```python
from build123d import *

# Parameters (mm, degrees)
SKETCH1_W           = 57
SKETCH1_H           = 52
BOSS_EXTRUDE1_DEPTH = 4
SKETCH3_W           = 37
SKETCH3_H           = 37
BOSS_EXTRUDE2_DEPTH = 3
SKETCH4_W           = 37
SKETCH4_H           = 37
BOSS_EXTRUDE3_DEPTH = 3
SKETCH6_R           = 1.5
BOSS_EXTRUDE4_DEPTH = 10
SKETCH6_6_R         = 1.5
BOSS_EXTRUDE6_DEPTH = 10
SKETCH8_W           = 4
SKETCH8_H           = 22
CUT_EXTRUDE1_DEPTH  = 11


with BuildPart() as part:
    # Sketch1 → Boss-Extrude1 (new body)
    with BuildSketch(Plane.XY):
        Rectangle(SKETCH1_W, SKETCH1_H)
    extrude(amount=BOSS_EXTRUDE1_DEPTH)

    # Sketch3 → Boss-Extrude2 (add)
    with BuildSketch(Plane.XY.offset(4)):
        with Locations((0, 7.5)):
            Rectangle(SKETCH3_W, SKETCH3_H)
    extrude(amount=BOSS_EXTRUDE2_DEPTH)

    # Sketch4 → Boss-Extrude3 (add)
    with BuildSketch(Plane(origin=(0, 0, 0), x_dir=(-1, 0, 0), z_dir=(0, 0, -1))):
        with Locations((0, 7.5)):
            Rectangle(SKETCH4_W, SKETCH4_H)
    extrude(amount=BOSS_EXTRUDE3_DEPTH)

    # Sketch6 → Boss-Extrude4 (add)
    with BuildSketch(Plane.XY):
        with Locations((14.91830134, 22.543210914)):
            Circle(SKETCH6_R)
        with Locations((14.91830134, -7.514403638)):
            Circle(SKETCH6_R)
    extrude(amount=-BOSS_EXTRUDE4_DEPTH)

    # Sketch6<6> → Boss-Extrude6 (add)
    with BuildSketch(Plane.XY):
        with Locations((-15.028807276, 22.543210914)):
            Circle(SKETCH6_6_R)
        with Locations((14.91830134, 22.543210914)):
            Circle(SKETCH6_6_R)
        with Locations((-15.028807276, -7.514403638)):
            Circle(SKETCH6_6_R)
        with Locations((14.91830134, -7.514403638)):
            Circle(SKETCH6_6_R)
    extrude(amount=-BOSS_EXTRUDE6_DEPTH)

    # Sketch8 → Cut-Extrude1 (cut, through all)
    with BuildSketch(Plane(origin=(0, 0, -3), x_dir=(-1, 0, 0), z_dir=(0, 0, -1))):
        with Locations((-15, 7.543210914)):
            Rectangle(SKETCH8_W, SKETCH8_H)
        with Locations((15, 7.543210914)):
            Rectangle(SKETCH8_W, SKETCH8_H)
    extrude(amount=-CUT_EXTRUDE1_DEPTH, mode=Mode.SUBTRACT)


solid = part.part
```
Part model, mm, in its own coordinate system. A direction names the side the tool comes from. Give positions to 0.01 mm unless a question says otherwise; leave off trailing zeros. Write each loop counter-clockwise with the first axis right and the second up, starting at its lowest first coordinate (ties: lowest second). Pieces come first, ordered by that corner, then holes. Notation, with made-up numbers: (-16.75, 1) -> (4.25, 1) arc R11 cw to (4.25, 15) -> close; hole circle Ø10 at (70.5, 67). An arc over 180 degrees is marked (long way). Put each result on its own line as item: value. Start each with the question number.
Item 1: Wall check: L1, parallel to Y at x = 16, z = 3.25; L2, parallel to Z at x = 24, y = -20; L3, parallel to Y at x = 1.5, z = -0.25. Give the ranges that are in metal, low to high. Write a range as [from, to].
Item 2: Cut at B-B (z = -0.75). List the corners of the cut face in (x, y).
Item 3: Cut at A-A (y = -0.5). List the corners of the cut face in (x, z), then the cut area to 3 significant figures.
Item 4: Which spindle directions (+Z, -Z, +X, -X, +Y, -Y) get a long thin tool onto all of the face, cutting with end or side? Do faces 1 (the face through (0, -11, -1)), 2 (the face through (0, -11, 5)), 3 (the face through (14.72, 24.03, -6.45)). Say none if no direction does.
Item 5: Pull direction Y, two halves, no side cores. Call faces 4 (the face through (0, -26, 2)), 5 (the face through (15, 23, -10)), 6 (the face through (-15, -3.457, 2)): pulls with the +Y half, pulls with the -Y half, needs draft (parallel to the pull), parting line crosses it, or undercut.
Item 6: Cut at D-D (x = 15.5). List the corners of the cut face in (y, z).
Item 7: Cut at C-C (x = -6.5). List the corners of the cut face in (y, z), then the cut area to 3 significant figures.
Item 8: Pin check, flat tips, straight feed: pin 1 Ø2.5 at (y, z) = (6, 5.5) entering from -X; pin 2 Ø3 at (x, y) = (6.5, -18.5) entering from -Z; pin 3 Ø0.9 at (x, z) = (3, -2) entering from -Y. Stop position of each tip, or through.
Answer list:
1. L1: y = [-26, -3.46], [18.54, 26]
1. L2: z = [0, 4]
1. L3: y = [-11, 26]
2. outline: (-18.5, -11) -> (18.5, -11) -> (18.5, 26) -> (-18.5, 26) -> close; hole (-17, -3.46) -> (-13, -3.46) -> (-13, 18.54) -> (-17, 18.54) -> close; hole (13, -3.46) -> (17, -3.46) -> (17, 18.54) -> (13, 18.54) -> close
3. outline: (-28.5, 0) -> (-18.5, 0) -> (-18.5, -3) -> (-17, -3) -> (-17, 7) -> (-18.5, 7) -> (-18.5, 4) -> (-28.5, 4) -> close; (-13, -3) -> (13, -3) -> (13, 7) -> (-13, 7) -> close; (17, -3) -> (18.5, -3) -> (18.5, 0) -> (28.5, 0) -> (28.5, 4) -> (18.5, 4) -> (18.5, 7) -> (17, 7) -> close
3. area: 370 mm2
4. face 1: -Z, +X, -X, -Y
4. face 2: +Z, +X, -X, -Y
4. face 3: -Z
5. face 4: pulls with the -Y half
5. face 5: needs draft
5. face 6: undercut
6. outline: (-26, 0) -> (-11, 0) -> (-11, -3) -> (-8.9, -3) -> (-8.9, -10) -> (-6.13, -10) -> (-6.13, -3) -> (-3.46, -3) -> (-3.46, 7) -> (-11, 7) -> (-11, 4) -> (-26, 4) -> close; (18.54, -3) -> (21.16, -3) -> (21.16, -10) -> (23.93, -10) -> (23.93, -3) -> (26, -3) -> (26, 7) -> (18.54, 7) -> close
7. outline: (-26, 0) -> (-11, 0) -> (-11, -3) -> (26, -3) -> (26, 7) -> (-11, 7) -> (-11, 4) -> (-26, 4) -> close
7. area: 430 mm2
8. pin 1: stops at x = -18.5
8. pin 2: stops at z = 0
8. pin 3: stops at y = -11
